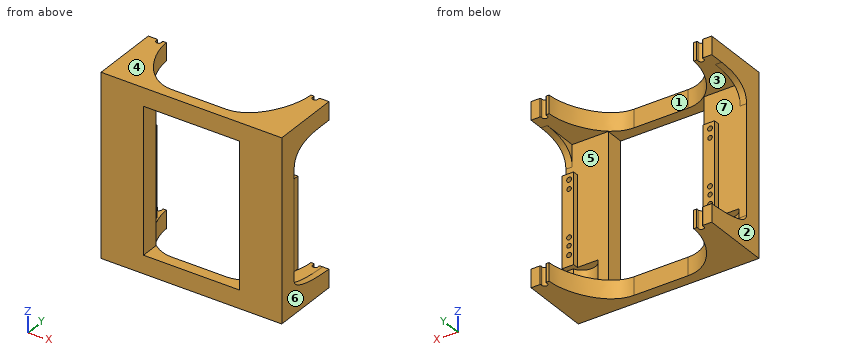
```python
from build123d import *

# Parameters (mm, degrees)
SKETCH_1_W          = 100
SKETCH_1_H          = 100
EXTRUDE_1_DEPTH     = 3
SKETCH_2_W          = 10
SKETCH_2_H          = 10
EXTRUDE_2_DEPTH     = 35
CUT_EXTRUDE_START   = -100
SKETCH_5_R          = 1.5
CUT_EXTRUDE_2_DEPTH = 100
FILLET_1_R          = 0.5
SKETCH_7_W          = 80
SKETCH_7_H          = 10
EXTRUDE_3_DEPTH     = 3
EXTRUDE_4_DEPTH     = 10
EXTRUDE_5_DEPTH     = 10
SKETCH_13_W         = 23.5
SKETCH_13_H         = 80
EXTRUDE_6_DEPTH     = 7
EXTRUDE_8_DEPTH     = 3.5
EXTRUDE_9_DEPTH     = 3.5
SKETCH_12_R         = 7.5
CUT_EXTRUDE_3_DEPTH = 13
SKETCH_14_W         = 6.37
SKETCH_14_H         = 49.8
SKETCH_14_R         = 1.35
SKETCH_14_R_2       = 1.25
EXTRUDE_7_DEPTH     = 3
SKETCH_3_W          = 53
SKETCH_3_H          = 80
CUT_EXTRUDE_1_DEPTH = 3


with BuildPart() as part:
    # 草图1 → 凸台-拉伸1 (new body)
    with BuildSketch(Plane(origin=(0, 0, 0), x_dir=(1, 0, 0), z_dir=(0, 1, 0))):
        Rectangle(SKETCH_1_W, SKETCH_1_H)
    extrude(amount=EXTRUDE_1_DEPTH)

    # 草图2 → 凸台-拉伸2 (add)
    with BuildSketch(Plane(origin=(0, 3, 0), x_dir=(1, 0, 0), z_dir=(0, 1, 0))):
        with Locations((45, 45)):
            Rectangle(SKETCH_2_W, SKETCH_2_H)
        with Locations((-45, 45)):
            Rectangle(SKETCH_2_W, SKETCH_2_H)
        with Locations((45, -45)):
            Rectangle(SKETCH_2_W, SKETCH_2_H)
        with Locations((-45, -45)):
            Rectangle(SKETCH_2_W, SKETCH_2_H)
    extrude(amount=EXTRUDE_2_DEPTH)

    # 草图5 → 切除-拉伸2 (cut)
    with BuildSketch(Plane(origin=(0, 0, -50), x_dir=(-1, 0, 0), z_dir=(0, 0, -1)).offset(CUT_EXTRUDE_START)):
        with Locations((-43.3, 36.8)):
            Circle(SKETCH_5_R)
        with Locations((43.3, 36.8)):
            Circle(SKETCH_5_R)
    extrude(amount=CUT_EXTRUDE_2_DEPTH, mode=Mode.SUBTRACT)

    # 圆角1
    fillet_1_edges = [part.edges().sort_by_distance(p)[0] for p in [
        (-44.2, 38, 45),
        (-42.4, 38, 45),
        (42.4, 38, 45),
        (44.2, 38, 45),
        (-42.4, 38, -45),
        (-44.2, 38, -45),
        (44.2, 38, -45),
        (42.4, 38, -45),
    ]]
    fillet(fillet_1_edges, radius=FILLET_1_R)

    # 草图7 → 凸台-拉伸3 (add)
    with BuildSketch(Plane(origin=(0, 3, 0), x_dir=(1, 0, 0), z_dir=(0, 1, 0))):
        with Locations((0, -45)):
            Rectangle(SKETCH_7_W, SKETCH_7_H)
        with Locations((0, 45)):
            Rectangle(SKETCH_7_W, SKETCH_7_H)
    extrude(amount=EXTRUDE_3_DEPTH)

    # 草图8 → 凸台-拉伸4 (add)
    with BuildSketch(Plane.XY.offset(50)):
        with BuildLine():
            Line((-40, 38), (-40, 6))
            Line((-40, 6), (-15, 6))
            add(Edge.make_bspline(
                [(-40, 38), (-40, 26.493596618), (-30.150326601, 6), (-15, 6)],
                knots=[0, 0, 0, 0, 1, 1, 1, 1], degree=3))
        make_face()
        with BuildLine():
            Line((40, 6), (15, 6))
            add(Edge.make_bspline(
                [(40, 38), (40, 26.493596618), (30.150326601, 6), (15, 6)],
                knots=[0, 0, 0, 0, 1, 1, 1, 1], degree=3))
            Line((40, 38), (40, 6))
        make_face()
    extrude(amount=-EXTRUDE_4_DEPTH)

    # 草图9 → 凸台-拉伸5 (add)
    with BuildSketch(Plane(origin=(0, 0, -50), x_dir=(-1, 0, 0), z_dir=(0, 0, -1))):
        with BuildLine():
            Line((-40, 6), (-15, 6))
            add(Edge.make_bspline(
                [(-15, 6), (-30.150326601, 6), (-40, 26.493596618), (-40, 38)],
                knots=[0, 0, 0, 0, 1, 1, 1, 1], degree=3))
            Line((-40, 38), (-40, 6))
        make_face()
        with BuildLine():
            Line((40, 6), (40, 38))
            add(Edge.make_bspline(
                [(40, 38), (40, 26.493596618), (30.150326601, 6), (15, 6)],
                knots=[0, 0, 0, 0, 1, 1, 1, 1], degree=3))
            Line((15, 6), (40, 6))
        make_face()
    extrude(amount=-EXTRUDE_5_DEPTH)

    # 草图13 → 凸台-拉伸6 (add)
    with BuildSketch(Plane(origin=(0, 3, 0), x_dir=(1, 0, 0), z_dir=(0, 1, 0))):
        with Locations((-38.25, 0)):
            Rectangle(SKETCH_13_W, SKETCH_13_H)
        with Locations((38.25, 0)):
            Rectangle(SKETCH_13_W, SKETCH_13_H)
    extrude(amount=EXTRUDE_6_DEPTH)

    # 草图17 → 凸台-拉伸8 (add)
    with BuildSketch(Plane(origin=(50, 0, 0), x_dir=(0, 0, -1), z_dir=(1, 0, 0))):
        with BuildLine():
            Line((32, 10), (40, 10))
            Line((40, 10), (40, 38))
            add(Edge.make_bspline(
                [(40, 38), (40, 35.102252049), (38.976100097, 10), (32, 10)],
                knots=[0, 0, 0, 0, 1, 1, 1, 1], degree=3))
        make_face()
        with BuildLine():
            Line((-40, 30), (-40, 10))
            Line((-40, 10), (-28, 10))
            add(Edge.make_bspline(
                [(-40, 30), (-40, 10), (-28, 10)],
                knots=[0, 0, 0, 1, 1, 1], degree=2))
        make_face()
    extrude(amount=-EXTRUDE_8_DEPTH)

    # 草图18 → 凸台-拉伸9 (add)
    with BuildSketch(Plane.ZY.offset(50)):
        with BuildLine():
            Line((40, 10), (40, 30))
            add(Edge.make_bspline(
                [(40, 30), (40, 10), (28, 10)],
                knots=[0, 0, 0, 1, 1, 1], degree=2))
            Line((28, 10), (40, 10))
        make_face()
        with BuildLine():
            Line((-40, 10), (-32, 10))
            add(Edge.make_bspline(
                [(-32, 10), (-38.976100097, 10), (-40, 35.102252049), (-40, 38)],
                knots=[0, 0, 0, 0, 1, 1, 1, 1], degree=3))
            Line((-40, 38), (-40, 10))
        make_face()
    extrude(amount=-EXTRUDE_9_DEPTH)

    # 草图12 → 切除-拉伸3 (cut)
    with BuildSketch(Plane.XY.offset(-40)):
        with Locations((-39, 13)):
            Circle(SKETCH_12_R)
        with Locations((39, 13)):
            Circle(SKETCH_12_R)
    extrude(amount=CUT_EXTRUDE_3_DEPTH, mode=Mode.SUBTRACT)

    # 草图14 → 凸台-拉伸7 (add)
    # profile 1 of 2: a face of its own
    with BuildSketch(Plane(origin=(0, 10, 0), x_dir=(1, 0, 0), z_dir=(0, 1, 0))):
        with Locations((-31.188863542, 2.1)):
            Rectangle(SKETCH_14_W, SKETCH_14_H)
        with Locations(Location((-31.873863542, 21, 0), (0, 0, 270))):
            Circle(SKETCH_14_R, mode=Mode.SUBTRACT)
        with Locations(Location((-31.873863542, 16, 0), (0, 0, 270))):
            Circle(SKETCH_14_R_2, mode=Mode.SUBTRACT)
        with Locations(Location((-31.873863542, 11.5, 0), (0, 0, 270))):
            Circle(SKETCH_14_R, mode=Mode.SUBTRACT)
        with Locations(Location((-31.873863542, -14.5, 0), (0, 0, 270))):
            Circle(SKETCH_14_R_2, mode=Mode.SUBTRACT)
        with Locations(Location((-31.873863542, -19.5, 0), (0, 0, 270))):
            Circle(SKETCH_14_R, mode=Mode.SUBTRACT)
    # profile 2 of 2: a face of its own
    with BuildSketch(Plane(origin=(0, 10, 0), x_dir=(1, 0, 0), z_dir=(0, 1, 0))):
        with Locations((46.811136458, 2.1)):
            Rectangle(SKETCH_14_W, SKETCH_14_H)
        with Locations(Location((46.126136458, 21, 0), (0, 0, 270))):
            Circle(SKETCH_14_R, mode=Mode.SUBTRACT)
        with Locations(Location((46.126136458, 16, 0), (0, 0, 270))):
            Circle(SKETCH_14_R_2, mode=Mode.SUBTRACT)
        with Locations(Location((46.126136458, 11.5, 0), (0, 0, 270))):
            Circle(SKETCH_14_R, mode=Mode.SUBTRACT)
        with Locations(Location((46.126136458, -14.5, 0), (0, 0, 270))):
            Circle(SKETCH_14_R_2, mode=Mode.SUBTRACT)
        with Locations(Location((46.126136458, -19.5, 0), (0, 0, 270))):
            Circle(SKETCH_14_R, mode=Mode.SUBTRACT)
    extrude(amount=EXTRUDE_7_DEPTH)

    # 草图3 → 切除-拉伸1 (cut)
    with BuildSketch(Plane(origin=(0, 3, 0), x_dir=(1, 0, 0), z_dir=(0, 1, 0))):
        Rectangle(SKETCH_3_W, SKETCH_3_H)
    extrude(amount=-CUT_EXTRUDE_1_DEPTH, mode=Mode.SUBTRACT)


solid = part.part
```
Here's how the part is built. I have some questions about the finished solid (model axes, mm). Face numbers are marked on the shaded views. A direction names the side the tool comes from. Coordinates: 2 decimals unless noted, no trailing zeros. Loops run counter-clockwise (first coordinate to the right, second up) from the corner with the lowest first, then second, coordinate; pieces in that order, holes last. Notation, with made-up numbers: (40, 73.5) - (55, 73.5) arc R6 ccw to (55, 84.5) - close; hole circle Ø8 at (66, 87). An arc over 180 degrees is marked (long way). Return JSON: item names as keys, results as strings. Group by question number.
Item 1: If we section it at C-C on x = -43.3: Write out the boundary of the cut face in (y, z).
Item 2: We'd pull the mould along Z, two halves only. Please class the marked faces 4, 5, 6 and 7: +Z half, -Z half, draft (parallel to the pull), parting line (faces both ways), or undercut.
Item 3: On a 3-axis mill with a long thin cutter (end or side, diameter ignored), from which of +Z, -Z, +X, -X, +Y, -Y can I reach the whole of each face in a straight line? I mean the marked faces 1, 2 and 3. Say none if no direction works.
Item 4: If we section it at D-D on y = 25: State how many separate pieces and enclosed holes the cut face has, and give its area (3 significant figures).
Item 5: I need wall thicknesses on line 1 (X direction, y = 11.1, z = -16); line 2 (X direction, y = 10.8, z = 19.5); line 3 (Z direction, x = -28.5, y = 11). Which ranges of each line are inside material? Lowest first, please. Write a range as from..to.
Item 6: Will these pins go through, and if not, where does the flat tip stop? P1, Ø1.4, axis at x = 46, z = 19.5, coming from the +Y side; P2, Ø3, axis at x = 46, z = 14.5, coming from the +Y side.
Calculated:
{
 "1": {"outline": "(0, -50) - (35.3, -50) - (35.3, -40) - (6.86, -40) - (6.86, -27) - (10, -27) - (10, 40) - (35.3, 40) - (35.3, 50) - (0, 50) - close"},
 "2": {"face 4": "+Z half", "face 5": "undercut", "face 6": "draft", "face 7": "undercut"},
 "3": {"face 1": "+Z, -Z, +Y", "face 2": "+Z, -Z, -X, +Y, -Y", "face 3": "+Y"},
 "4": {"separate pieces": "4", "enclosed holes": "0", "area": "527 mm^2"},
 "5": {"line 1": "x = -34.37..-33.12, -30.62..-28, 43.63..44.88, 47.38..50", "line 2": "x = -34.37..-33.22, -30.52..-28, 43.63..44.78, 47.48..50", "line 3": "z = -50..-40, -27..22.8, 40..50"},
 "6": {"P1": "stops at y = 10", "P2": "stops at y = 13"}
}
